```python
from build123d import *

# Parameters (mm, degrees)
SKETCH1_R               = 5.5
BOSS_EXTRUDE1_DEPTH     = 7
CUT_EXTRUDE3_DEPTH      = 7
SKETCH3_R               = 4.5
BOSS_EXTRUDE2_DEPTH     = 4
SKETCH4_R               = 1.5
CUT_EXTRUDE4_DEPTH      = 6
CUT_EXTRUDE4_DEPTH_BACK = 6
SKETCH5_R               = 2.5
CUT_EXTRUDE5_DEPTH      = 12


with BuildPart() as part:
    # Sketch1 → Boss-Extrude1 (new body)
    with BuildSketch(Plane.XY):
        Circle(SKETCH1_R)
    extrude(amount=BOSS_EXTRUDE1_DEPTH)

    # Sketch2 → Cut-Extrude3 (cut)
    with BuildSketch(Plane.XY.offset(7)):
        Polygon((0, 4.75), (-0.5, 5.75), (0.5, 5.75), align=None)
        Polygon((0.824828844, 4.677836827), (0.506073145, 5.749468669), (1.490880898, 5.575820491), align=None)
        Polygon((1.624595681, 4.463539949), (1.496769514, 5.574242641), (2.436462135, 5.232222498), align=None)
        Polygon((2.375, 4.113620668), (2.441987298, 5.229646072), (3.308012702, 4.729646072), align=None)
        Polygon((3.053241146, 3.638711105), (3.313006534, 4.726149353), (4.079050977, 4.083361743), align=None)
        Polygon((3.638711105, 3.053241146), (4.083361743, 4.079050977), (4.726149353, 3.313006534), align=None)
        Polygon((4.113620668, 2.375), (4.729646072, 3.308012702), (5.229646072, 2.441987298), align=None)
        Polygon((4.463539949, 1.624595681), (5.232222498, 2.436462135), (5.574242641, 1.496769514), align=None)
        Polygon((4.677836827, 0.824828844), (5.575820491, 1.490880898), (5.749468669, 0.506073145), align=None)
        Polygon((4.75, 0), (5.75, 0.5), (5.75, -0.5), align=None)
        Polygon((4.677836827, -0.824828844), (5.749468669, -0.506073145), (5.575820491, -1.490880898), align=None)
        Polygon((4.463539949, -1.624595681), (5.574242641, -1.496769514), (5.232222498, -2.436462135), align=None)
        Polygon((4.113620668, -2.375), (5.229646072, -2.441987298), (4.729646072, -3.308012702), align=None)
        Polygon((3.638711105, -3.053241146), (4.726149353, -3.313006534), (4.083361743, -4.079050977), align=None)
        Polygon((3.053241146, -3.638711105), (4.079050977, -4.083361743), (3.313006534, -4.726149353), align=None)
        Polygon((2.375, -4.113620668), (3.308012702, -4.729646072), (2.441987298, -5.229646072), align=None)
        Polygon((1.624595681, -4.463539949), (2.436462135, -5.232222498), (1.496769514, -5.574242641), align=None)
        Polygon((0.824828844, -4.677836827), (1.490880898, -5.575820491), (0.506073145, -5.749468669), align=None)
        Polygon((0, -4.75), (0.5, -5.75), (-0.5, -5.75), align=None)
        Polygon((-0.824828844, -4.677836827), (-0.506073145, -5.749468669), (-1.490880898, -5.575820491), align=None)
        Polygon((-1.624595681, -4.463539949), (-1.496769514, -5.574242641), (-2.436462135, -5.232222498), align=None)
        Polygon((-2.375, -4.113620668), (-2.441987298, -5.229646072), (-3.308012702, -4.729646072), align=None)
        Polygon((-3.053241146, -3.638711105), (-3.313006534, -4.726149353), (-4.079050977, -4.083361743), align=None)
        Polygon((-3.638711105, -3.053241146), (-4.083361743, -4.079050977), (-4.726149353, -3.313006534), align=None)
        Polygon((-4.113620668, -2.375), (-4.729646072, -3.308012702), (-5.229646072, -2.441987298), align=None)
        Polygon((-4.463539949, -1.624595681), (-5.232222498, -2.436462135), (-5.574242641, -1.496769514), align=None)
        Polygon((-4.677836827, -0.824828844), (-5.575820491, -1.490880898), (-5.749468669, -0.506073145), align=None)
        Polygon((-4.75, 0), (-5.75, -0.5), (-5.75, 0.5), align=None)
        Polygon((-4.677836827, 0.824828844), (-5.749468669, 0.506073145), (-5.575820491, 1.490880898), align=None)
        Polygon((-4.463539949, 1.624595681), (-5.574242641, 1.496769514), (-5.232222498, 2.436462135), align=None)
        Polygon((-4.113620668, 2.375), (-5.229646072, 2.441987298), (-4.729646072, 3.308012702), align=None)
        Polygon((-3.638711105, 3.053241146), (-4.726149353, 3.313006534), (-4.083361743, 4.079050977), align=None)
        Polygon((-3.053241146, 3.638711105), (-4.079050977, 4.083361743), (-3.313006534, 4.726149353), align=None)
        Polygon((-2.375, 4.113620668), (-3.308012702, 4.729646072), (-2.441987298, 5.229646072), align=None)
        Polygon((-1.624595681, 4.463539949), (-2.436462135, 5.232222498), (-1.496769514, 5.574242641), align=None)
        Polygon((-0.824828844, 4.677836827), (-1.490880898, 5.575820491), (-0.506073145, 5.749468669), align=None)
    extrude(amount=-CUT_EXTRUDE3_DEPTH, mode=Mode.SUBTRACT)

    # Sketch3 → Boss-Extrude2 (add)
    with BuildSketch(Plane.XY.offset(7)):
        Circle(SKETCH3_R)
    extrude(amount=BOSS_EXTRUDE2_DEPTH)

    # Sketch4 → Cut-Extrude4 (cut, two sides)
    with BuildSketch(Plane(origin=(0, 0, 0), x_dir=(0, 0, -1), z_dir=(1, 0, 0))) as cut_extrude4_sk:
        with Locations((-9, 0)):
            Circle(SKETCH4_R)
    extrude(amount=CUT_EXTRUDE4_DEPTH, mode=Mode.SUBTRACT)
    extrude(cut_extrude4_sk.sketch, amount=-CUT_EXTRUDE4_DEPTH_BACK, mode=Mode.SUBTRACT)

    # Sketch5 → Cut-Extrude5 (cut)
    with BuildSketch(Plane.XY.offset(11)):
        Circle(SKETCH5_R)
    extrude(amount=-CUT_EXTRUDE5_DEPTH, mode=Mode.SUBTRACT)


solid = part.part
```
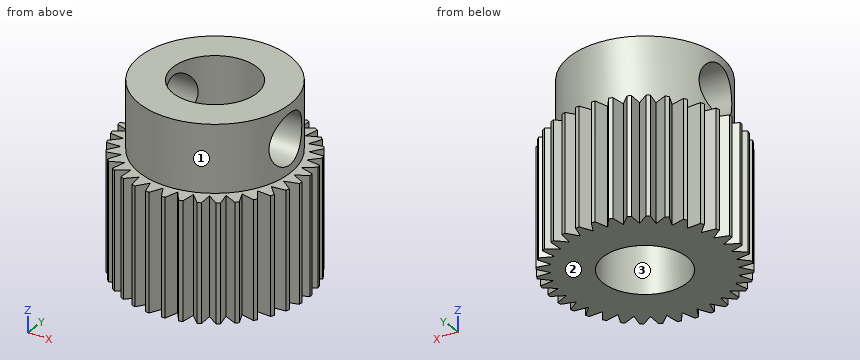
Source: CAD feature listing. Evaluate the final solid. Frame: model axes, mm. Face numbers are marked on the shaded views. Coordinates: 2 decimals unless noted, no trailing zeros. Write each loop counter-clockwise with the first axis right and the second up, starting at its lowest first coordinate (ties: lowest second). Pieces come first, ordered by that corner, then holes. Notation, with made-up numbers: (-37, 31.5) -> (18, 31.5) arc R7 cw to (18, 43.5) -> close; hole circle Ø6 at (-27.5, 73.25). An arc over 180 degrees is marked (long way). Return JSON: item names as keys, results as strings. Group by question number.
1) Mould query, pull axis Y, two halves, no side actions, for the marked faces 1, 2 and 3. Classes: +Y half, -Y half, draft (parallel to the pull), parting line (faces both ways), or undercut.
2) Contact query for flat-ended pins moving along their axis: P1, Ø2, axis at x = 1.5, z = 3.5, coming from the +Y side; P2, Ø1.5, axis at y = 3, z = 2, coming from the +X side. Output: stop coordinate, or through.
3) Ray query, line 1 along Z through (x, y) = (2.8, 0); line 2 along X through (y, z) = (5.25, 5); line 3 along Y through (x, z) = (-1, 8). Return the intervals inside material, ascending.
4) Section query A-A, the plane z = 9. Return loops of the section in (x, y).
From the geometry:
{
 "1": {"face 1": "parting line", "face 2": "draft", "face 3": "undercut"},
 "2": {"P1": "y = 5.48", "P2": "x = 5.02"},
 "3": {"line 1": "0 to 7.5, 10.5 to 11", "line 2": "-1.53 to -1.25, -0.65 to -0.25, 0.25 to 0.65, 1.25 to 1.53", "line 3": "-4.39 to -2.29, 2.29 to 4.39"},
 "4": {"outline": "(-4.24, -1.5) arc R4.5 ccw to (4.24, -1.5) -> (2, -1.5) arc R2.5 cw to (-2, -1.5) -> close; (-4.24, 1.5) -> (-2, 1.5) arc R2.5 cw to (2, 1.5) -> (4.24, 1.5) arc R4.5 ccw to start"}
}
